Input: part model. Units: mm. Frame: model coordinates. A direction names the side the tool comes from. Give positions to 0.01 mm unless a question says otherwise; leave off trailing zeros. Write each loop counter-clockwise with the first axis right and the second up, starting at its lowest first coordinate (ties: lowest second). Pieces come first, ordered by that corner, then holes. Notation, with made-up numbers: (48, 49.5) - (70, 49.5) arc R14 ccw to (70, 57.5) - close; hole circle Ø6 at (8, -20.5). An arc over 180 degrees is marked (long way). Use a Markdown table: item, result. Add a question column.
1. Material intervals for probe 1 along Y at (x, z) = (42.5, 1.7); probe 2 along Y at (x, z) = (27.5, 0.7); probe 3 along Y at (x, z) = (28, 0.15), sorted ascending.
2. Section query C-C, the plane x = -20.5. Return loops of the section in (y, z), plus the area to 3 significant figures.
3. Section query A-A, the plane y = -57.15. Return loops of the section in (x, z), plus the area to 3 significant figures.
4. Set-up query: faces 1 (the flat face through (22, 6.35, 1)), 2 (the flat face through (1.524, -27, 1)). Return all of +Z, -Z, +X, -X, +Y, -Y with unobstructed straight access to the full face (end or side cutting, diameter ignored); none if empty.
5. Mould query, pull axis X, two halves, no side actions, for faces 3 (the flat face through (13, -45, 2.54)), 4 (the flat face through (53.34, -45, 1)), 5 (the flat face through (20, -72.136, 1)). Classes: released by +X, released by -X, zero draft, split by the parting line, or undercut.
6. Section query B-B, the plane z = 1. Count the separate pieces of the cut face and the enclosed holes in it, plus the area to 3 significant figures.
7. Pin query (flat end, axial travel): pin 1 (0.8 mm diameter, centred on y = -45, z = 1, fed in from -X); pin 2 (3 mm diameter, centred on x = 18.8, y = -86.54, fed in from -Z); pin 3 (2 mm diameter, centred on x = -17.45, y = -57.15, fed in from +Z). Return the tip coordinate at first contact, or that it passes through.
```python
from build123d import *

# Parameters (mm, degrees)
SKETCH1_R           = 1.27
BOSS_EXTRUDE1_DEPTH = 2.54
SKETCH5_W           = 8.382
SKETCH5_H           = 8.382
SKETCH5_W_2         = 2.794
SKETCH5_H_2         = 43.434
CUT_EXTRUDE1_DEPTH  = 3.54
SKETCH7_R           = 1.27
CUT_EXTRUDE3_DEPTH  = 3.54
SKETCH8_W           = 12.7
SKETCH8_H           = 2.54
SKETCH8_W_2         = 2.54
SKETCH8_H_2         = 12.7
CUT_EXTRUDE4_DEPTH  = 3.54


with BuildPart() as part:
    # Sketch1 → Boss-Extrude1 (new body)
    with BuildSketch(Plane.XY):
        with BuildLine():
            Line((-3.314058103, 6.35), (48.26, 6.35))
            ThreePointArc((48.26, 6.35), (51.852102448, 4.862102448), (53.34, 1.27))
            Line((53.34, 1.27), (53.34, -92.71))
            ThreePointArc((53.34, -92.71), (51.852102448, -96.302102448), (48.26, -97.79))
            Line((48.26, -97.79), (16.846989059, -97.79))
            ThreePointArc((16.846989059, -97.79), (15.638688158, -97.644208035), (14.499741809, -97.215200367))
            Line((14.499741809, -97.215200367), (-16.7505185, -80.933552139))
            ThreePointArc((-16.7505185, -80.933552139), (-18.059258376, -79.955412607), (-18.989802686, -78.61241436))
            Line((-18.989802686, -78.61241436), (-28.309569459, -59.040904135))
            ThreePointArc((-28.309569459, -59.040904135), (-28.795802898, -57.127870198), (-28.51617555, -55.173917704))
            Line((-28.51617555, -55.173917704), (-8.107195629, 2.952923842))
            ThreePointArc((-8.107195629, 2.952923842), (-6.251501454, 5.414614163), (-3.314058103, 6.35))
        make_face()
        with Locations((48.0822, 2.286)):
            Circle(SKETCH1_R, mode=Mode.SUBTRACT)
        with Locations((-3.718687848, 1.651)):
            Circle(SKETCH1_R, mode=Mode.SUBTRACT)
        with Locations((-25.012261453, -59.761967182)):
            Circle(SKETCH1_R, mode=Mode.SUBTRACT)
    extrude(amount=BOSS_EXTRUDE1_DEPTH)

    # Sketch5 → Cut-Extrude1 (cut, through all)
    with BuildSketch(Plane(origin=(0, 0, 0), x_dir=(-1, 0, 0), z_dir=(0, 0, -1))):
        with Locations((-36.83, -17.78)):
            Rectangle(SKETCH5_W, SKETCH5_H)
        with Locations((-39.37, -45.72)):
            Rectangle(SKETCH5_W, SKETCH5_H)
        with Locations((-36.83, -27.94)):
            Rectangle(SKETCH5_W, SKETCH5_H)
        with Locations((-41.91, -64.77)):
            Rectangle(SKETCH5_W, SKETCH5_H)
        with Locations((-41.91, -83.82)):
            Rectangle(SKETCH5_W, SKETCH5_H)
        with Locations((-22.098, -17.78)):
            Rectangle(SKETCH5_W, SKETCH5_H)
        with Locations((-22.098, -27.94)):
            Rectangle(SKETCH5_W, SKETCH5_H)
        with Locations((-23.622, -45.72)):
            Rectangle(SKETCH5_W, SKETCH5_H)
        with Locations((-25.146, -64.77)):
            Rectangle(SKETCH5_W, SKETCH5_H)
        with Locations((-15.367, -26.543)):
            Rectangle(SKETCH5_W_2, SKETCH5_H_2)
        with Locations((-0.127, -26.543)):
            Rectangle(SKETCH5_W_2, SKETCH5_H_2)
    extrude(amount=-CUT_EXTRUDE1_DEPTH, mode=Mode.SUBTRACT)

    # Sketch7 → Cut-Extrude3 (cut, through all)
    with BuildSketch(Plane.XY.offset(2.54)):
        with Locations((44.2976, -2.4892)):
            Circle(SKETCH7_R)
        with Locations((1.6002, -2.4384)):
            Circle(SKETCH7_R)
        with Locations((-17.4498, -57.15)):
            Circle(SKETCH7_R)
        with Locations((-10.5918, -71.3486)):
            Circle(SKETCH7_R)
        with Locations((18.796, -86.5378)):
            Circle(SKETCH7_R)
    extrude(amount=-CUT_EXTRUDE3_DEPTH, mode=Mode.SUBTRACT)

    # Sketch8 → Cut-Extrude4 (cut, through all)
    with BuildSketch(Plane.XY.offset(2.54)):
        with Locations((29.972, -83.312)):
            Rectangle(SKETCH8_W, SKETCH8_H)
        with Locations((20.066, -78.486)):
            Rectangle(SKETCH8_W_2, SKETCH8_H_2)
        with Locations((13.208, -81.026)):
            Rectangle(SKETCH8_W_2, SKETCH8_H_2)
        with Locations((5.588, -78.486)):
            Rectangle(SKETCH8_W_2, SKETCH8_H_2)
    extrude(amount=-CUT_EXTRUDE4_DEPTH, mode=Mode.SUBTRACT)


solid = part.part
```
Result sheet:
| question | item | result |
|---|---|---|
| 1 | probe 1 | y = -97.79 to -88.01, -79.63 to -68.96, -60.58 to -49.91, -41.53 to 6.35 |
| 1 | probe 2 | y = -97.79 to -84.58, -82.04 to -68.96, -60.58 to -49.91, -41.53 to 6.35 |
| 1 | probe 3 | y = -97.79 to -84.58, -82.04 to -68.96, -60.58 to 6.35 |
| 2 | outline | (-75.44, 0) - (-32.34, 0) - (-32.34, 2.54) - (-75.44, 2.54) - close |
| 2 | area | 109 mm² |
| 3 | outline | (-28.79, 0) - (-18.72, 0) - (-18.72, 2.54) - (-28.79, 2.54) - close; (-16.18, 0) - (53.34, 0) - (53.34, 2.54) - (-16.18, 2.54) - close |
| 3 | area | 202 mm² |
| 4 | face 1 | +Z, -Z, +X, -X, +Y |
| 4 | face 2 | +Z, -Z |
| 5 | face 3 | zero draft |
| 5 | face 4 | released by +X |
| 5 | face 5 | undercut |
| 6 | separate pieces | 1 |
| 6 | enclosed holes | 23 |
| 6 | area | 6,210 mm² |
| 7 | pin 1 | stops at x = -25.08 |
| 7 | pin 2 | stops at z = 0 |
| 7 | pin 3 | passes through |
